Could you check a few things on this model? Use its own coordinates, in mm. Face numbers are marked on the shaded views. Give positions to 0.01 mm unless a question says otherwise; leave off trailing zeros. Order: outer loops, then holes, each group sorted by start corner. A loop starts at its lowest first (then second) coordinate and runs counter-clockwise, first axis right, second up.
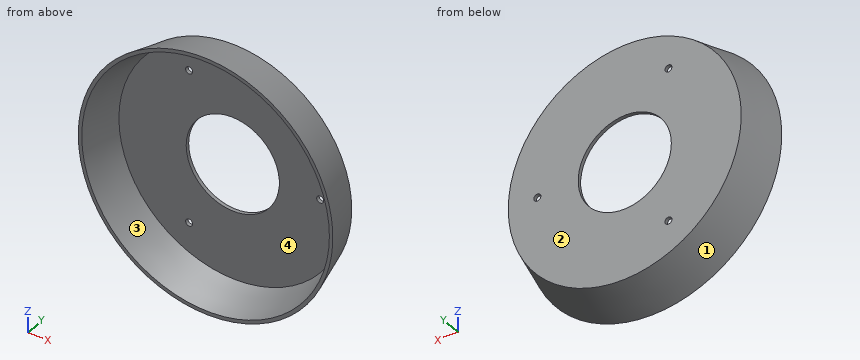
from build123d import *

# Parameters (mm, degrees)
SKETCH001_R     = 1.5
HOLE_DEPTH      = 25
COPYSKETCH002_R = 20
POCKET_DEPTH    = 5


with BuildPart() as part:
    # Sketch → Revolution (revolve)
    with BuildSketch(Plane.XY):
        Polygon((-54.6463, 0), (-53.1463, 0), (-48.887192, 16.5), (0, 16.5), (0, 18), (-50, 18), align=None)
    revolve(axis=Axis((0, 0, 0), (0, 1, 0)))

    # Sketch001 (on Face4 of Revolution) → Hole (cut)
    with BuildSketch(Plane(origin=(0, 18, 0), x_dir=(-1, 0, 0), z_dir=(0, 1, 0))):
        with Locations((-37.5, 0)):
            Circle(SKETCH001_R)
        with Locations((18.75, 32.475953)):
            Circle(SKETCH001_R)
        with Locations((18.75, -32.475953)):
            Circle(SKETCH001_R)
        Circle(SKETCH001_R)
    extrude(amount=-HOLE_DEPTH, mode=Mode.SUBTRACT)

    # CopySketch002 → Pocket (cut)
    with BuildSketch(Plane(origin=(0, 18, 0), x_dir=(-1, 0, 0), z_dir=(0, 1, 0))):
        Circle(COPYSKETCH002_R)
    extrude(amount=-POCKET_DEPTH, mode=Mode.SUBTRACT)


solid = part.part
Item 1: Imagine slicing it at A-A on x = 0. List the corners of the cut face in (y, z) for me.
Findings:
outline: (0, -54.65) - (18, -50) - (18, -20) - (16.5, -20) - (16.5, -48.89) - (0, -53.15) - close; (0, 53.15) - (16.5, 48.89) - (16.5, 20) - (18, 20) - (18, 50) - (0, 54.65) - close
Item 2: Imagine slicing it at B-B on z = 0. List the corners of the cut face in (x, y) for me, then the cut area to 3 significant figures.
Findings:
outline: (-54.65, 0) - (-53.15, 0) - (-48.89, 16.5) - (-20, 16.5) - (-20, 18) - (-50, 18) - close; (20, 16.5) - (36, 16.5) - (36, 18) - (20, 18) - close; (39, 16.5) - (48.89, 16.5) - (53.15, 0) - (54.65, 0) - (50, 18) - (39, 18) - close
area: 136 mm2
Item 3: We'd pull the mould along Z, two halves only. Please class the marked faces 1, 2, 3 and 4: +Z half, -Z half, draft (parallel to the pull), parting line (faces both ways), or undercut.
Findings:
face 1: parting line
face 2: draft
face 3: undercut
face 4: undercut
Item 4: Imagine slicing it at C-C on y = 8. List the corners of the cut face in (x, z) for me, then the cut area to 3 significant figures.
Findings:
outline: circle Ø105.16 at (0, 0); hole circle Ø102.16 at (0, 0)
area: 488 mm2
Item 5: Please list where these lines run through material, in increasing order: line 1 along Y through (x, z) = (-6, 34.5); line 2 along Z through (x, y) = (-29, 1.25); line 3 along X through (y, z) = (9.5, -11).
Findings:
line 1: y = 16.5 to 18
line 2: z = -45.94 to -44.15, 44.15 to 45.94
line 3: x = -51.02 to -49.49, 49.49 to 51.02
Item 6: For pin 1 (3.5 mm diameter, centred on x = -18.75, z = 32.48, fed in from +Y); pin 2 (3 mm diameter, centred on y = 5, z = -19, fed in from +X); pin 3 (8 mm diameter, centred on x = 10, z = 19, fed in from -Y); pin 4 (1 mm diameter, centred on y = 11.5, z = -19, fed in from -X), each with a flat end and sliding along its axis, tell me the tip position at first contact or that it passes through.
Findings:
pin 1: stops at y = 18
pin 2: stops at x = 50.55
pin 3: stops at y = 16.5
pin 4: stops at x = -48.3
